```python
from build123d import *

# Parameters (mm, degrees)
SKETCH_1_W          = 94
SKETCH_1_H          = 88
EXTRUDE_1_DEPTH     = 4
SKETCH_2_W          = 20
SKETCH_2_H          = 20
CUT_EXTRUDE_1_DEPTH = 65.505813691
FILLET_1_R          = 3
SKETCH_3_R          = 2.5
CUT_EXTRUDE_2_DEPTH = 65.505813691
SKETCH_4_R          = 1.5
CUT_EXTRUDE_3_DEPTH = 65.505813691


with BuildPart() as part:
    # 草图1 → 凸台-拉伸1 (new body)
    with BuildSketch(Plane.XY):
        Rectangle(SKETCH_1_W, SKETCH_1_H)
    extrude(amount=EXTRUDE_1_DEPTH)

    # 草图2 → 切除-拉伸1 (cut, through all)
    with BuildSketch(Plane.XY.offset(4)):
        with Locations((-37, 34)):
            Rectangle(SKETCH_2_W, SKETCH_2_H)
        with Locations((37, 34)):
            Rectangle(SKETCH_2_W, SKETCH_2_H)
    extrude(amount=-CUT_EXTRUDE_1_DEPTH, mode=Mode.SUBTRACT)

    # 圆角1
    fillet_1_edges = [part.edges().sort_by_distance(p)[0] for p in [
        (-47, 24, 2),
        (-27, 44, 2),
        (-27, 24, 2),
        (27, 44, 2),
        (47, 24, 2),
        (27, 24, 2),
    ]]
    fillet(fillet_1_edges, radius=FILLET_1_R)

    # 草图3 → 切除-拉伸2 (cut, through all)
    with BuildSketch(Plane.XY.offset(4)):
        with Locations((-15, -1)):
            Circle(SKETCH_3_R)
        with Locations((15, -1)):
            Circle(SKETCH_3_R)
        with Locations((15, -31)):
            Circle(SKETCH_3_R)
        with Locations((-15, -31)):
            Circle(SKETCH_3_R)
    extrude(amount=-CUT_EXTRUDE_2_DEPTH, mode=Mode.SUBTRACT)

    # 草图4 → 切除-拉伸3 (cut, through all)
    with BuildSketch(Plane.XY.offset(4)):
        with Locations((-15, 36.5)):
            Circle(SKETCH_4_R)
        with Locations((39.5, 14)):
            Circle(SKETCH_4_R)
        with Locations((39.5, -36)):
            Circle(SKETCH_4_R)
        with Locations(Location((15, 36.5, 0), (0, 0, 180))):
            Circle(SKETCH_4_R)
        with Locations(Location((-39.5, -36, 0), (0, 0, 180))):
            Circle(SKETCH_4_R)
        with Locations(Location((-39.5, 14, 0), (0, 0, 180))):
            Circle(SKETCH_4_R)
    extrude(amount=-CUT_EXTRUDE_3_DEPTH, mode=Mode.SUBTRACT)


solid = part.part
```
Geometry check sheet. Reference: the model listing, model coordinates, mm. A direction names the side the tool comes from. Give positions to 0.01 mm unless a question says otherwise; leave off trailing zeros. Loops run counter-clockwise (first coordinate to the right, second up) from the corner with the lowest first, then second, coordinate; pieces in that order, holes last. Notation, with made-up numbers: M 48.5,46.5 L 78.5,46.5 A29 cw 78.5,71.5 Z; hole C 17,47.25 d3. An arc over 180 degrees is marked long. Answer as CSV lines item,"result".
Item 1: Release check for a two-part mould opening along X. For faces 4 (the cylindrical face through (-46.14, 23.1, 1.97)), 5 (the cylindrical face through (46.1, 23.14, 1.97)), 6 (the cylindrical face through (38.3, -36.9, 2)), 7 (the flat face through (-1, 1, 4)) record: pulls with the +X half, pulls with the -X half, needs draft (parallel to the pull), parting line crosses it, or undercut.
Values:
face 4,"pulls with the -X half"
face 5,"pulls with the +X half"
face 6,"undercut"
face 7,"needs draft"
Item 2: Cross-section at A-A on x = 39.5. Record the cut outline in (y, z).
Values:
outline,"M -44,0 L -37.5,0 L -37.5,4 L -44,4 Z; M -34.5,0 L 12.5,0 L 12.5,4 L -34.5,4 Z; M 15.5,0 L 24,0 L 24,4 L 15.5,4 Z"
Item 3: Access from +Z, -Z, +X, -X, +Y, -Y to the whole of each face (thin tool, end or side, straight path). Record for faces 1 (the cylindrical face through (-16.2, 35.6, 2)), 2 (the flat face through (37, 24, 2)), 3 (the flat face through (-37, 24, 2)).
Values:
face 1,"+Z, -Z"
face 2,"+Z, -Z, +X, +Y"
face 3,"+Z, -Z, -X, +Y"
Item 4: Cross-section at D-D on x = 15. Record the cut outline in (y, z), and give its area (3 significant figures).
Values:
outline,"M -44,0 L -33.5,0 L -33.5,4 L -44,4 Z; M -28.5,0 L -3.5,0 L -3.5,4 L -28.5,4 Z; M 1.5,0 L 35,0 L 35,4 L 1.5,4 Z; M 38,0 L 44,0 L 44,4 L 38,4 Z"
area,"300 mm²"
Item 5: Cross-section at B-B on y = -1. Record the cut outline in (x, z), and give its area (3 significant figures).
Values:
outline,"M -47,0 L -17.5,0 L -17.5,4 L -47,4 Z; M -12.5,0 L 12.5,0 L 12.5,4 L -12.5,4 Z; M 17.5,0 L 47,0 L 47,4 L 17.5,4 Z"
area,"336 mm²"
Item 6: Depth check by flat-ended pin: P1, Ø1, axis at x = 34, z = 2.5, coming from the +Y side; P2, Ø2, axis at y = 29, z = 2.5, coming from the +X side. Enter the tip coordinate at first touch or a pass-through.
Values:
P1,"stops at y = 24"
P2,"stops at x = 27"
Item 7: Cross-section at C-C on z = 1.5. Count the separate pieces of the cut face and the enclosed holes in it, and give its area (3 significant figures).
Values:
separate pieces,"1"
enclosed holes,"10"
area,"7,350 mm²"
Item 8: Material ranges on line 1 (Y direction, x = -39.5, z = 1.9); line 2 (Y direction, x = -15, z = 2.65); line 3 (X direction, y = 1, z = 1.3), recorded low to high.
Values:
line 1,"y = -44 to -37.5, -34.5 to 12.5, 15.5 to 24"
line 2,"y = -44 to -33.5, -28.5 to -3.5, 1.5 to 35, 38 to 44"
line 3,"x = -47 to -16.5, -13.5 to 13.5, 16.5 to 47"
